Geometry check sheet. Reference: the model listing, model coordinates, mm. Round coordinates to 2 decimals unless told otherwise and drop trailing zeros. Loops run counter-clockwise (first coordinate to the right, second up) from the corner with the lowest first, then second, coordinate; pieces in that order, holes last. Notation, with made-up numbers: M 7,58.25 L 21,58.25 A24 cw 21,90.25 Z; hole C 35,47.25 d2. An arc over 180 degrees is marked long. Write item = value, one per line.
from build123d import *

# Parameters (mm, degrees)
SKETCH_1_R      = 75
EXTRUDE_1_DEPTH = 5
HOLE_WIZARD_2_D = 5.1


with BuildPart() as part:
    # 草图1 → 凸台-拉伸1 (new body)
    with BuildSketch(Plane(origin=(0, 0, 0), x_dir=(1, 0, 0), z_dir=(0, 1, 0))):
        with Locations(Location((0, 0, 0), (0, 0, 270))):
            Circle(SKETCH_1_R)
    extrude(amount=EXTRUDE_1_DEPTH)

    # 孔2 (through all)
    with Locations(Plane.XZ):
        with Locations((34.79, -34.79), (34.79, 34.79), (-34.79, -34.79), (-34.79, 34.79)):
            Hole(HOLE_WIZARD_2_D / 2)


solid = part.part
(1) Sectioned sample at D-D on x = 54. Record the cut outline in (y, z).
Result set:
outline = M 0,-52.05 L 5,-52.05 L 5,52.05 L 0,52.05 Z
(2) Sectioned sample at A-A on y = 1.8. Record the cut outline in (x, z), then the cut area to 3 significant figures.
Result set:
outline = C 0,0 d150; hole C -34.79,-34.79 d5.1; hole C -34.79,34.79 d5.1; hole C 34.79,-34.79 d5.1; hole C 34.79,34.79 d5.1
area = 17,600 mm2
(3) Material ranges on line 1 along X through (y, z) = (1.9, 36); line 2 along Z through (x, y) = (34.79, 3.6); line 3 along Z through (x, y) = (23, 2.5), recorded low to high. Write a range as from..to.
Result set:
line_1 = -65.8..-37.03, -32.55..32.55, 37.03..65.8
line_2 = -66.44..-37.34, -32.24..32.24, 37.34..66.44
line_3 = -71.39..71.39
(4) Sectioned sample at B-B on x = 34.79. Record the cut outline in (y, z).
Result set:
outline = M 0,-66.44 L 5,-66.44 L 5,-37.34 L 0,-37.34 Z; M 0,-32.24 L 5,-32.24 L 5,32.24 L 0,32.24 Z; M 0,37.34 L 5,37.34 L 5,66.44 L 0,66.44 Z
(5) Sectioned sample at C-C on z = 34.79. Record the cut outline in (x, y), then the cut area to 3 significant figures.
Result set:
outline = M -66.44,0 L -37.34,0 L -37.34,5 L -66.44,5 Z; M -32.24,0 L 32.24,0 L 32.24,5 L -32.24,5 Z; M 37.34,0 L 66.44,0 L 66.44,5 L 37.34,5 Z
area = 613 mm2
(6) Release check for a two-part mould opening along X. For faces 1 (the cylindrical face through (37.338, 2.535, 34.902)), 2 (the cylindrical face through (-45.636, 2.465, -59.517)), 3 (the flat face through (1, 5, -1)) record: released by +X, released by -X, zero draft, split by the parting line, or undercut.
Result set:
face_1 = undercut
face_2 = split by the parting line
face_3 = zero draft
(7) Depth check by flat-ended pin: pin 1 Ø1 at (y, z) = (1, -30.5) entering from +X; pin 2 Ø3 at (y, z) = (2, -0.5) entering from +X; pin 3 Ø3 at (x, y) = (44.5, 2.5) entering from -Z; pin 4 Ø6 at (x, z) = (-34.79, 34.79) entering from -Y. Enter the tip coordinate at first touch or a pass-through.
Result set:
pin_1 = 68.74
pin_2 = 75
pin_3 = -61.45
pin_4 = 0
